Input: dimensioned drawing with shaded views. Units: mm. Origin: part minimum x, y, z. A direction names the side the tool comes from. Give positions to 0.01 mm unless a question says otherwise; leave off trailing zeros. Write each loop counter-clockwise with the first axis right and the second up, starting at its lowest first coordinate (ties: lowest second). Pieces come first, ordered by that corner, then holes.
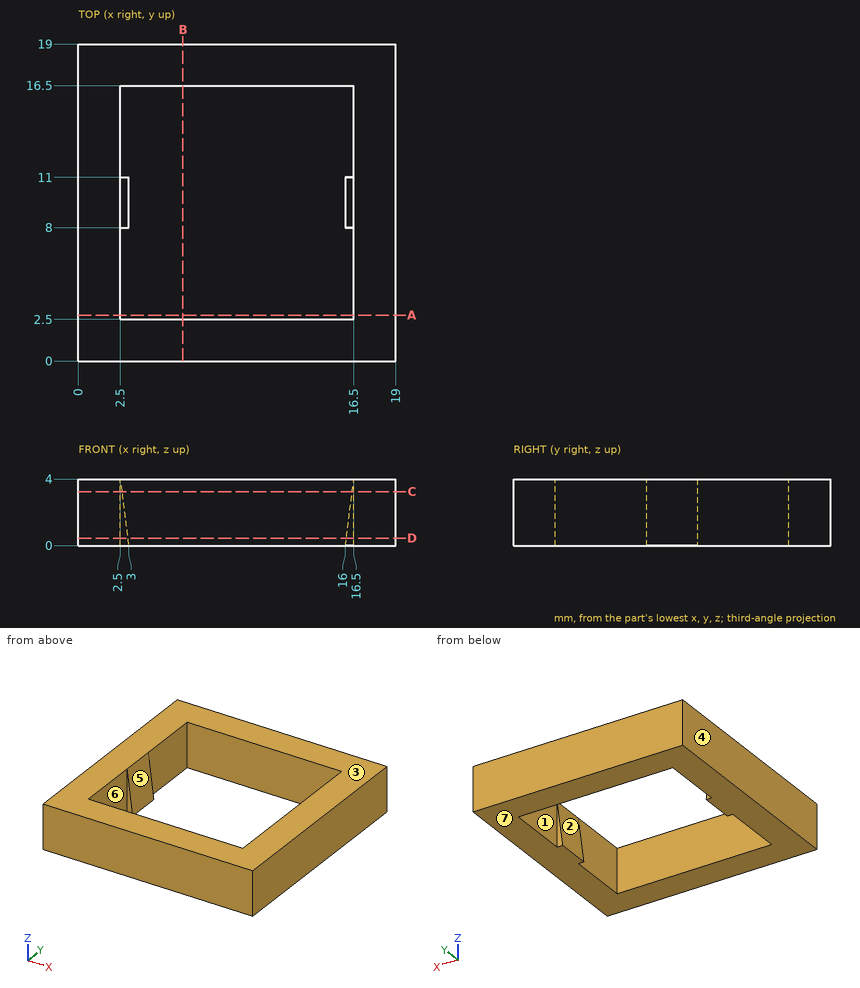
Item 1: Pin query (flat end, axial travel): pin 1 Ø5 at (x, y) = (17, 16) entering from -Z. Return the tip coordinate at first contact, or that it passes through.
Found:
pin 1: stops at z = 0
Item 2: Section C-C, the plane z = 3.25. Return the cut outline in (x, y), plus the area to 3 significant figures.
Found:
outline: (0, 0) - (19, 0) - (19, 19) - (0, 19) - close; hole (2.5, 2.5) - (16.5, 2.5) - (16.5, 8) - (16.41, 8) - (16.41, 11) - (16.5, 11) - (16.5, 16.5) - (2.5, 16.5) - (2.5, 11) - (2.59, 11) - (2.59, 8) - (2.5, 8) - close
area: 166 mm2
Item 3: Pull-direction query (X, two-part tool) for the marked faces 4, 5, 6 and 7; classes: +X half, -X half, draft (parallel to the pull), parting line (faces both ways), or undercut.
Found:
face 4: -X half
face 5: undercut
face 6: undercut
face 7: draft
Item 4: Section D-D, the plane z = 0.45. Return the cut outline in (x, y), plus the area to 3 significant figures.
Found:
outline: (0, 0) - (19, 0) - (19, 19) - (0, 19) - close; hole (2.5, 2.5) - (16.5, 2.5) - (16.5, 8) - (16.06, 8) - (16.06, 11) - (16.5, 11) - (16.5, 16.5) - (2.5, 16.5) - (2.5, 11) - (2.94, 11) - (2.94, 8) - (2.5, 8) - close
area: 168 mm2
Item 5: Reachability of the marked faces 1, 2 and 3 from +Z, -Z, +X, -X, +Y, -Y: full face, straight path, thin tool, end or side. Return the list, or none.
Found:
face 1: +Z, -Z
face 2: +Z
face 3: +Z, +X, -X, +Y, -Y
Item 6: Section A-A, the plane y = 2.75. Return the cut outline in (x, z).
Found:
outline: (0, 0) - (2.5, 0) - (2.5, 4) - (0, 4) - close; (16.5, 0) - (19, 0) - (19, 4) - (16.5, 4) - close
Item 7: Line query: L1, parallel to X at y = 3.5, z = 0.6; L2, parallel to X at y = 9, z = 1 (3 decimals). Output: solid intervals per line, ascending.
Found:
L1: x = 0 to 2.5, 16.5 to 19
L2: x = 0 to 2.875, 16.125 to 19
